Check sheet for the modelled part. Datum: model origin and axes. Units: mm. A direction names the side the tool comes from. Coordinates: 2 decimals unless noted, no trailing zeros.
1. Set-up check for faces 1 (the flat face through (-88.6, -7, -2.1)), 2 (the flat face through (-2, -9, 1)): record each of +Z, -Z, +X, -X, +Y, -Y from which the full face is reachable in a straight line by a thin tool's end or side.
2. Thickness scan on line 1 (X direction, y = -6.25, z = 29); line 2 (X direction, y = -6.25, z = 31.5); line 3 (Y direction, x = -92, z = 56). Record the ranges inside material, lowest first.
3. Cross-section at A-A (y = -1.5). Count the separate pieces of the cut face and the enclosed holes in it, then the cut area to 3 significant figures.
4. Gauge pin test, flat ends, axial feed: pin 1 Ø4 at (y, z) = (-7.5, 23) entering from +X; pin 2 Ø3 at (x, y) = (120, -7.5) entering from -Z; pin 3 Ø3 at (x, y) = (-43.5, -2.5) entering from +Z; pin 4 Ø1.5 at (x, z) = (113, 1.5) entering from +Y. Record the tip position at first contact, or that the pin passes through.
5. Draft check along X on faces 3 (the cylindrical face through (93.68, -4.48, -81.99)), 4 (the flat face through (-2, 0, 1)), 5 (the cylindrical face through (-152.537, -4.479, 1.277)). Enter one of: released by +X, released by -X, zero draft, split by the parting line, or undercut.
```python
from build123d import *

# Parameters (mm, degrees)
F1_DEPTH = 9
F3_R     = 3
F4_DEPTH = 4
F6_D     = 4


with BuildPart() as f1:
    # F0 (on Front) → F1 (new body)
    with BuildSketch(Plane.XZ):
        with BuildLine():
            ThreePointArc((-53.1497258364, 79.5460974403), (-94.56723042, 81.6982905812), (-129.933253949, 60.0352806103))
            ThreePointArc((-129.933253949, 60.0352806103), (-152.5456475155, 0.3641086136), (-130.4114859728, -59.4861044443))
            ThreePointArc((-130.4114859728, -59.4861044443), (-94.8267257051, -81.5334878267), (-53.0234392177, -79.3317802685))
            add(Edge.make_bspline(
                [(-53.0234392177, -79.3317802685), (-48.6608082648, -77.7082088333), (-24.6397852476, -70.4889476448), (23.7505923387, -70.5665306527), (48.2937092789, -77.8753902125), (52.9987360366, -79.6127570647)],
                knots=[0.192962823, 0.192962823, 0.192962823, 0.192962823, 0.2940919494, 0.7017955969, 0.810107416, 0.810107416, 0.810107416, 0.810107416], degree=3))
            ThreePointArc((52.9987360366, -79.6127570647), (94.2508745118, -81.8498183409), (129.5801249251, -60.4351636118))
            ThreePointArc((129.5801249251, -60.4351636118), (152.5456748781, 0.3572045933), (129.1035766867, 60.9674062841))
            ThreePointArc((129.1035766867, 60.9674062841), (93.9984455084, 82.0081589209), (53.1289942993, 79.8237907218))
            add(Edge.make_bspline(
                [(-53.1497258364, 79.5460974403), (-48.7515954924, 77.9273408187), (-24.7040875075, 70.7832354564), (23.8166554522, 70.8602953804), (48.3873163026, 78.0925624494), (53.1289942993, 79.8237907218)],
                knots=[0.1918397391, 0.1918397391, 0.1918397391, 0.1918397391, 0.2939558653, 0.7019159659, 0.8112404118, 0.8112404118, 0.8112404118, 0.8112404118], degree=3))
        make_face()
    extrude(amount=F1_DEPTH)

    # F3
    f3_edges = [f1.edges().sort_by_distance(p)[0] for p in [
        (-94.56723, -9, 81.698291),
        (0.004128, -9, 71.956269),
        (93.998446, -9, 82.008159),
        (152.545675, -9, 0.357205),
        (94.250875, -9, -81.849818),
        (0.002547, -9, -71.678393),
        (-94.826726, -9, -81.533488),
        (-152.545648, -9, 0.364109),
        (-94.56723, 0, 81.698291),
    ]]
    fillet(f3_edges, radius=F3_R)

    # F2 (on face) → F4 (cut)
    with BuildSketch(Plane.XZ.offset(9)):
        Polygon((94.4679220363, 66.3983235541), (64.8748605741, -70.4382604186), (73.6714981152, -72.3406715126), (103.2645595774, 64.4959124601), align=None)
        Polygon((-76.2725546155, -72.0010940176), (-67.4092848384, -70.4382604186), (-91.7200297117, 67.4348250031), (-100.5832994888, 65.8719914041), align=None)
    extrude(amount=-F4_DEPTH, mode=Mode.SUBTRACT)

    # F6 (through all)
    with Locations(Plane.XZ.offset(9)):
        with Locations((-90.0739783819, 32.1851368482), (-77.9186059453, -36.7514058626), (76.6714447102, -37.1803199724), (91.4679754413, 31.2379720139)):
            Hole(F6_D / 2)


solid = f1.part
```
Data:
1. face 1: -Y
1. face 2: +Z, -Z, +X, -X, -Y
2. line 1: x = -147.79 to -94.08, -84.94 to 86.38, 95.59 to 147.79
2. line 2: x = -146.91 to -94.52, -85.38 to 86.92, 96.13 to 146.91
2. line 3: y = -5 to 0
3. separate pieces: 1
3. enclosed holes: 4
3. area: 43,200 mm2
4. pin 1: stops at x = 149.98
4. pin 2: stops at z = -70.24
4. pin 3: stops at z = 76.91
4. pin 4: stops at y = 0
5. face 3: undercut
5. face 4: zero draft
5. face 5: released by -X
